Autodesk Inventor part; units mm, degrees
ref_plane "Work Plane1" through (29, 0, 0) normal (0, -1, 0) x (1, 0, 0)
ref_plane "YZ Plane" through (0, 0, 0) normal (1, 0, 0) x (0, 1, 0)
ref_plane "XZ Plane" through (0, 0, 0) normal (0, 1, 0) x (-1, 0, 0)
sketch "Skizze1" plane through (0, 0, 0) normal (0, 0, 1) x (1, 0, 0)
  line L0 (0.2267, 0) -> (40, 0)
  line L1 (40, 0) -> (40, 6)
  line L2 (40, 6) -> (5.25, 6)
  line L3 (5.25, 6) -> (4.1764, 6)
  line L4 (4.1764, 6) -> (0, 6)
  line L5 (0, 6) -> (0, 10.5)
  line L6 (0, 10.5) -> (-6.6, 10.5)
  line L7 (-6.6, 10.5) -> (-6.6, 4.6188)
  line L8 (-6.6, 4.6188) -> (-2.44, 4.6188)
  line L9 (-2.44, 4.6188) -> (0.2267, 0)
  line L10 (-15.92, 0) -> (49.32, 0)
  line L11 (0, -2.1) -> (0, 12.6)
  line L12 (5.25, 6) -> (0, 6) construction
  dimension "d1" = 34.75
  dimension "d2" = 1.0736
  dimension "d3" = 6.6
  dimension "d4" = 4.16
  dimension "d5" = 60
  dimension "d6" = 12
  dimension "d7" = 12
  dimension "d8" = 9.2376
  dimension "d9" = 21
  dimension "d26" = 40
revolve "Körper" add sketch "Skizze1" angle 360 about axis through (0.2267, 0, 0) along (1, 0, 0) contours L9 L11 L4 L3 L2 L1 L0 | L9 L8 L7 L6 L5 L11
sketch "Skizze2" plane through (-6.6, 0, 0) normal (-1, 0, 0) x (0, 0, 1)
  circle A0 centre (0, 0) radius 4.6188
  line L0 (0, -14.7) -> (0, 14.7)
  line L1 (-14.7, 0) -> (14.7, 0)
  line L2 (4.6188, 0) -> (2.3094, -4)
  line L3 (2.3094, -4) -> (-2.3094, -4)
  line L4 (-2.3094, -4) -> (-4.6188, 0)
  line L5 (-4.6188, 0) -> (-2.3094, 4)
  line L6 (-2.3094, 4) -> (2.3094, 4)
  line L7 (2.3094, 4) -> (4.6188, 0)
extrude "Loch" add sketch "Skizze2" against normal up to next contours L7 A0 | A0 L2 | L6 L0 A0 | A0 L0 L3 | L0 L6 A0 | A0 L3 L0 | L4 A0 | A0 L5
fillet "Rundung1" radius 4.97 1 edges at (-6.6, -10.5, 0)
thread "Gewinde"
chamfer "Fase1" distance 1.0735 distance2 1.0735 1 edges at (40, -6, 0) measured on face at (40, -2.3028, -0.7984)
ref_plane "Work Plane1" through (29, 0, 0) normal (0, -1, 0) x (1, 0, 0)
fillet "Rundung2" radius 1.1 1 edges at (0, -6, 0)
equation "\"d1\" = GEL"
equation "\"d3\" = KOH"
equation "\"d4\" = INTI"
equation "\"d6\" = GD"
equation "\"d7\" = BDM"
equation "\"d8\" = 1.1547 * SW"
equation "\"d9\" = KOD"
equation "\"d26\" = NLG"
equation "\"d17\" = RR"
equation "\"d13\" = GEL"
equation "\"d15\" = -0.5 * SPD + 0.5 * GD"
equation "\"d16\" = GUL"
equation "\"d30\" = R"
equation "\"GD\" = NND"
equation "\"NLG\" = 40"
equation "\"GEL\" = 34.75"
equation "\"KOD\" = 21"
equation "\"KOH\" = 6.6"
equation "\"INTI\" = 4.16"
equation "\"GAL\" = 0.61345 * PTC"
equation "\"GUL\" = 0.61345 * PTC"
equation "\"BDM\" = NND"
equation "\"SW\" = 8"
equation "\"RR\" = 4.97"
equation "\"SPD\" = NND - 1.2269 * PTC"
equation "\"R\" = 1.1"
equation "\"TOA\" = 30deg"
equation "\"GD1\" = THREADDIA - 1.2269 * PTC"
equation "\"THREADDIA\" = 12"
equation "\"PTC\" = 1.75"
equation "\"NND\" = 12"
equation "\"KOH1\" = 1.63"
equation "\"E0\" = 9.149"
properties part number "ISO 7380-1 - M12 x 40" material "Stahl"
CAD build for the part. Positions are in the model's coordinates, mm. A direction names the side the tool comes from. Coordinates: 2 decimals unless noted, no trailing zeros. Write each loop counter-clockwise with the first axis right and the second up, starting at its lowest first coordinate (ties: lowest second). Pieces come first, ordered by that corner, then holes. Notation, with made-up numbers: M 44.5,30 L 101.5,30 A14 ccw 101.5,44 Z; hole C 78,51 d6. An arc over 180 degrees is marked long. Return JSON: item names as keys, results as strings.
Item 1: Drop flat-ended pins along their axis: pin 1 Ø5 at (x, z) = (20.5, 4) entering from -Y; pin 2 Ø1.5 at (x, z) = (17.5, -5.5) entering from -Y; pin 3 Ø12 at (x, z) = (11.5, 7) entering from -Y. Give the stop position or say it passes through.
Findings below:
{"pin 1": "stops at y = -5.81", "pin 2": "stops at y = -3.67", "pin 3": "stops at y = -5.92"}
Item 2: Probe line 1 (Y direction, x = -1, z = -0.25); line 2 (Y direction, x = 30, z = -4.75); line 3 (Z direction, x = 20, y = 0.75). List the from-to ranges inside material, lowest first. Write a range as from..to.
Findings below:
{"line 1": "y = -10.5..-2.11, 2.11..10.5", "line 2": "y = -3.67..3.67", "line 3": "z = -5.95..5.95"}
Item 3: Which spindle directions (+Z, -Z, +X, -X, +Y, -Y) get a long thin tool onto all of the face, cutting with end or side? Do faces 1 (the flat face through (40, 0, 0)), 2 (the flat face through (0, 2, -7)), 3 (the flat face through (-4.37, -1.97, 3.48)). Say none if no direction does.
Findings below:
{"face 1": "+Z, -Z, +X, +Y, -Y", "face 2": "+X", "face 3": "-X"}
Item 4: Two-plate mould, pull along Z, no slides. Class faces 4 (the flat face through (-4.37, 1.97, -3.48)), 5 (the flat face through (-4.373, 2.028, 3.448)), 6 (the cylindrical face through (-0.8, 10, -3.2)), 7 (the flat face through (-6.6, -2, -4)): +Z half, -Z half, draft (parallel to the pull), parting line (faces both ways), or undercut.
Findings below:
{"face 4": "undercut", "face 5": "undercut", "face 6": "parting line", "face 7": "draft"}
Item 5: Slice it at A-A, the plane x = 7. Write the cut outline in (y, z).
Findings below:
{"outline": "C 0,0 d12"}
